Check sheet for the modelled part. Datum: model origin and axes. Units: mm. Face numbers are marked on the shaded views. Round coordinates to 2 decimals unless told otherwise and drop trailing zeros. Write each loop counter-clockwise with the first axis right and the second up, starting at its lowest first coordinate (ties: lowest second). Pieces come first, ordered by that corner, then holes.
from build123d import *

# Parameters (mm, degrees)
SKETCH1_R               = 7.5
BOSS_EXTRUDE1_DEPTH     = 50.5
SKETCH2_W               = 2
SKETCH2_H               = 5.5
CUT_EXTRUDE1_DEPTH      = 1.5
SKETCH3_W               = 5.5
SKETCH3_H               = 2
CUT_EXTRUDE2_DEPTH      = 1.5
SKETCH4_W               = 5.5
SKETCH4_H               = 2
CUT_EXTRUDE3_DEPTH      = 1.5
SKETCH5_W               = 5.5
SKETCH5_H               = 3.854101966
CUT_EXTRUDE4_DEPTH      = 6.25
MIRROR3_COPY_1_SKETCH_W = 2
MIRROR3_COPY_1_SKETCH_H = 5.5
MIRROR3_COPY_1_DEPTH    = 1.5
MIRROR3_COPY_2_SKETCH_W = 5.5
MIRROR3_COPY_2_SKETCH_H = 2
MIRROR3_COPY_2_DEPTH    = 1.5
MIRROR3_COPY_3_SKETCH_W = 5.5
MIRROR3_COPY_3_SKETCH_H = 2
MIRROR3_COPY_3_DEPTH    = 1.5
MIRROR3_COPY_4_SKETCH_W = 5.5
MIRROR3_COPY_4_SKETCH_H = 3.854101966
MIRROR3_COPY_4_DEPTH    = 6.25


with BuildPart() as part:
    # Sketch1 → Boss-Extrude1 (new body)
    with BuildSketch(Plane.XY):
        with BuildLine():
            Line((0, 9), (39, 9))
            ThreePointArc((39, 9), (46.794228634, 4.5), (46.794228634, -4.5))
            Line((46.794228634, -4.5), (37.044228634, -21.387495374))
            ThreePointArc((37.044228634, -21.387495374), (33.75, -24.681724008), (29.25, -25.887495374))
            Line((29.25, -25.887495374), (9.75, -25.887495374))
            ThreePointArc((9.75, -25.887495374), (5.25, -24.681724008), (1.955771366, -21.387495374))
            Line((1.955771366, -21.387495374), (-7.794228634, -4.5))
            ThreePointArc((-7.794228634, -4.5), (-7.794228634, 4.5), (0, 9))
        make_face()
        with Locations(Location((0, 0, 0), (0, 0, 180))):
            Circle(SKETCH1_R, mode=Mode.SUBTRACT)
        with Locations(Location((9.75, -16.887495374, 0), (0, 0, 180))):
            Circle(SKETCH1_R, mode=Mode.SUBTRACT)
        with Locations(Location((19.5, 0, 0), (0, 0, 180))):
            Circle(SKETCH1_R, mode=Mode.SUBTRACT)
        with Locations(Location((39, 0, 0), (0, 0, 180))):
            Circle(SKETCH1_R, mode=Mode.SUBTRACT)
        with Locations(Location((29.25, -16.887495374, 0), (0, 0, 180))):
            Circle(SKETCH1_R, mode=Mode.SUBTRACT)
    extrude(amount=BOSS_EXTRUDE1_DEPTH)

    # Sketch2 → Cut-Extrude1 (cut)
    with BuildSketch(Plane(origin=(37.044228634, -21.387495374, 0), x_dir=(0, 0, -1), z_dir=(0.8660254037844384, -0.5000000000000007, 0))):
        with Locations((-5.25, 9.75)):
            Rectangle(SKETCH2_W, SKETCH2_H)
    cut_extrude1 = extrude(amount=-CUT_EXTRUDE1_DEPTH, mode=Mode.SUBTRACT)

    # Sketch3 → Cut-Extrude2 (cut)
    with BuildSketch(Plane(origin=(0, 9, 0), x_dir=(1, 0, 0), z_dir=(0, 1, 0))):
        with Locations((29.25, -5.25)):
            Rectangle(SKETCH3_W, SKETCH3_H)
    cut_extrude2 = extrude(amount=-CUT_EXTRUDE2_DEPTH, mode=Mode.SUBTRACT)

    # Sketch4 → Cut-Extrude3 (cut)
    with BuildSketch(Plane.XZ.offset(25.887495374)):
        with Locations((19.5, 5.25)):
            Rectangle(SKETCH4_W, SKETCH4_H)
    cut_extrude3 = extrude(amount=-CUT_EXTRUDE3_DEPTH, mode=Mode.SUBTRACT)

    # Sketch5 → Cut-Extrude4 (cut)
    with BuildSketch(Plane(origin=(0, 0, 0), x_dir=(-1, 0, 0), z_dir=(0, 0, -1))):
        with Locations((-29.25, 5.822949017)):
            Rectangle(SKETCH5_W, SKETCH5_H)
        with Locations((-19.5, -22.710444391)):
            Rectangle(SKETCH5_W, SKETCH5_H)
        Polygon((-38.873946668, -8.010126843), (-36.123946668, -12.773266564), (-39.461696879, -14.700317547), (-42.211696879, -9.937177826), align=None)
    cut_extrude4 = extrude(amount=-CUT_EXTRUDE4_DEPTH, mode=Mode.SUBTRACT)

    # Mirror2: Cut-Extrude1, Cut-Extrude2, Cut-Extrude3, Cut-Extrude4 across plane
    add(cut_extrude1.mirror(Plane.ZY.offset(-19.5)), mode=Mode.SUBTRACT)
    add(cut_extrude2.mirror(Plane.ZY.offset(-19.5)), mode=Mode.SUBTRACT)
    add(cut_extrude3.mirror(Plane.ZY.offset(-19.5)), mode=Mode.SUBTRACT)
    add(cut_extrude4.mirror(Plane.ZY.offset(-19.5)), mode=Mode.SUBTRACT)

    # Mirror3: Cut-Extrude1, Cut-Extrude2, Cut-Extrude3, Cut-Extrude4 across plane
    add(cut_extrude1.mirror(Plane(origin=(0, 0, 25.25), x_dir=(1, 0, 0), z_dir=(0, 0, -1))), mode=Mode.SUBTRACT)
    add(cut_extrude2.mirror(Plane(origin=(0, 0, 25.25), x_dir=(1, 0, 0), z_dir=(0, 0, -1))), mode=Mode.SUBTRACT)
    add(cut_extrude3.mirror(Plane(origin=(0, 0, 25.25), x_dir=(1, 0, 0), z_dir=(0, 0, -1))), mode=Mode.SUBTRACT)
    add(cut_extrude4.mirror(Plane(origin=(0, 0, 25.25), x_dir=(1, 0, 0), z_dir=(0, 0, -1))), mode=Mode.SUBTRACT)

    # Mirror3 copy 1 sketch → Mirror3 copy 1 (cut)
    with BuildSketch(Plane(origin=(1.955771366, -21.387495374, 50.5), x_dir=(0, 0, 1), z_dir=(-0.8660254037844384, -0.5000000000000007, 1.2779807689605148e-15))):
        with Locations((-5.25, 9.75)):
            Rectangle(MIRROR3_COPY_1_SKETCH_W, MIRROR3_COPY_1_SKETCH_H)
    extrude(amount=-MIRROR3_COPY_1_DEPTH, mode=Mode.SUBTRACT)

    # Mirror3 copy 2 sketch → Mirror3 copy 2 (cut)
    with BuildSketch(Plane(origin=(39, 9, 50.5), x_dir=(-1, 0, 0), z_dir=(0, 1, 0))):
        with Locations((29.25, -5.25)):
            Rectangle(MIRROR3_COPY_2_SKETCH_W, MIRROR3_COPY_2_SKETCH_H)
    extrude(amount=-MIRROR3_COPY_2_DEPTH, mode=Mode.SUBTRACT)

    # Mirror3 copy 3 sketch → Mirror3 copy 3 (cut)
    with BuildSketch(Plane(origin=(39, -25.887495374, 50.5), x_dir=(-1, 0, 0), z_dir=(0, -1, 0))):
        with Locations((19.5, 5.25)):
            Rectangle(MIRROR3_COPY_3_SKETCH_W, MIRROR3_COPY_3_SKETCH_H)
    extrude(amount=-MIRROR3_COPY_3_DEPTH, mode=Mode.SUBTRACT)

    # Mirror3 copy 4 sketch → Mirror3 copy 4 (cut)
    with BuildSketch(Plane(origin=(39, 0, 50.5), x_dir=(1, 0, 0), z_dir=(0, 0, 1))):
        with Locations((-29.25, 5.822949017)):
            Rectangle(MIRROR3_COPY_4_SKETCH_W, MIRROR3_COPY_4_SKETCH_H)
        with Locations((-19.5, -22.710444391)):
            Rectangle(MIRROR3_COPY_4_SKETCH_W, MIRROR3_COPY_4_SKETCH_H)
        Polygon((-38.873946668, -8.010126843), (-36.123946668, -12.773266564), (-39.461696879, -14.700317547), (-42.211696879, -9.937177826), align=None)
    extrude(amount=-MIRROR3_COPY_4_DEPTH, mode=Mode.SUBTRACT)


solid = part.part
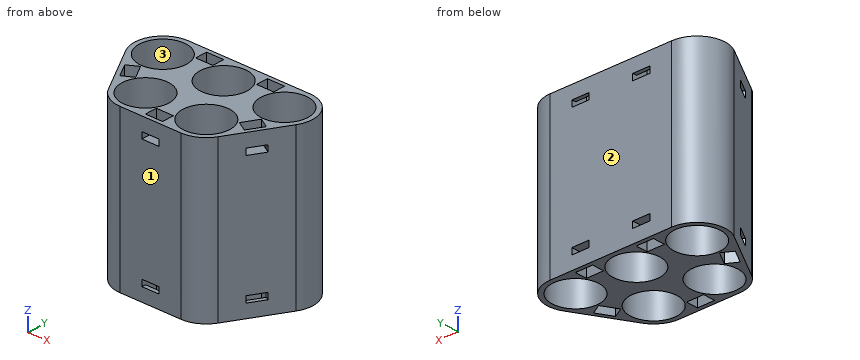
1. Scan lines: line 1 along Z through (x, y) = (-2.5, -11.5); line 2 along Y through (x, z) = (29.25, 19.5); line 3 along X through (y, z) = (-6, 4). Record each from-to range of solid material in increasing order.
2. Sectioned sample at B-B, the plane x = 19.5. Enter the section's corners in (y, z), plus the area to 3 significant figures.
3. Sectioned sample at D-D, the plane z = 38.5. Enter the section's corners in (x, y), plus the area to 3 significant figures.
4. Sectioned sample at C-C, the plane y = -23.5. Enter the section's corners in (x, z).
5. Go/stop test with flat-tipped pins: pin 1 (2 mm diameter, centred on x = 33.5, y = -5, fed in from +Z); pin 2 (1 mm diameter, centred on y = -9, z = 7.5, fed in from +X); pin 3 (6 mm diameter, centred on y = -16, z = 21.5, fed in from +X); pin 4 (1.5 mm diameter, centred on x = 28, y = 5.5, fed in from +Z). Record where each tip stops, or that it passes through.
6. Sectioned sample at A-A, the plane y = 0. Enter the section's corners in (x, z).
7. Release check for a two-part mould opening along Y. For the marked faces 1, 2 and 3 record: released by +Y, released by -Y, zero draft, split by the parting line, or undercut.
Computed values:
1. line 1: z = 0 to 4.25, 6.25 to 44.25, 46.25 to 50.5
1. line 2: y = -25.89 to -24.39, -9.39 to 9
1. line 3: x = -6.93 to -4.5, 4.5 to 15, 24 to 34.5, 43.5 to 45.93
2. outline: (-25.89, 0) - (-24.64, 0) - (-24.64, 4.25) - (-25.89, 4.25) - close; (-25.89, 6.25) - (-20.78, 6.25) - (-20.78, 0) - (-7.5, 0) - (-7.5, 50.5) - (-20.78, 50.5) - (-20.78, 44.25) - (-25.89, 44.25) - close; (-25.89, 46.25) - (-24.64, 46.25) - (-24.64, 50.5) - (-25.89, 50.5) - close; (7.5, 0) - (9, 0) - (9, 50.5) - (7.5, 50.5) - close
2. area: 951 mm2
3. outline: (-7.79, -4.5) - (1.96, -21.39) arc R9 ccw to (9.75, -25.89) - (29.25, -25.89) arc R9 ccw to (37.04, -21.39) - (46.79, -4.5) arc R9 ccw to (39, 9) - (0, 9) arc R9 ccw to start; hole circle Ø15 at (0, 0); hole circle Ø15 at (9.75, -16.89); hole circle Ø15 at (19.5, 0); hole circle Ø15 at (29.25, -16.89); hole circle Ø15 at (39, 0)
3. area: 742 mm2
4. outline: (3.64, 0) - (6.21, 0) - (6.21, 50.5) - (3.64, 50.5) - close; (13.29, 0) - (16.75, 0) - (16.75, 6.25) - (22.25, 6.25) - (22.25, 0) - (25.71, 0) - (25.71, 50.5) - (22.25, 50.5) - (22.25, 44.25) - (16.75, 44.25) - (16.75, 50.5) - (13.29, 50.5) - close; (32.79, 0) - (35.36, 0) - (35.36, 50.5) - (32.79, 50.5) - close
5. pin 1: stops at z = 50.5
5. pin 2: stops at x = 44.48
5. pin 3: stops at x = 41.89
5. pin 4: stops at z = 44.25
6. outline: (-9, 0) - (-7.5, 0) - (-7.5, 50.5) - (-9, 50.5) - close; (7.5, 0) - (12, 0) - (12, 50.5) - (7.5, 50.5) - close; (27, 0) - (31.5, 0) - (31.5, 50.5) - (27, 50.5) - close; (46.5, 0) - (48, 0) - (48, 50.5) - (46.5, 50.5) - close
7. face 1: released by -Y
7. face 2: released by +Y
7. face 3: undercut
